from build123d import *

# Parameters (mm, degrees)
SKETCH_1_W                   = 15.864971157
SKETCH_1_H                   = 12.5
EXTRUDE_1_DEPTH              = 10
EXTRUDE_2_DEPTH              = 7.5
EXTRUDE_3_DEPTH              = 7.5
HOLE_WIZARD_M3_1_D           = 3.3
HOLE_WIZARD_M3_1_DEPTH       = 9.8
HOLE_WIZARD_M3_1_CBORE_D     = 6
HOLE_WIZARD_M3_1_CBORE_DEPTH = 0.8
HOLE_WIZARD_M3_1_TIP         = 0.991420021
HOLE_WIZARD_M3_2_D           = 3.4
HOLE_WIZARD_M3_2_CBORE_D     = 6.5
HOLE_WIZARD_M3_2_CBORE_DEPTH = 3.5
FILLET_1_R                   = 3
CHAMFER_1_SIZE               = 1.5
FILLET_2_R                   = 2


with BuildPart() as part:
    # 草图1 → 凸台-拉伸1 (new body)
    with BuildSketch(Plane(origin=(0, 5, 0), x_dir=(1, 0, 0), z_dir=(0, 1, 0))):
        with Locations((16.367514422, -6.25)):
            Rectangle(SKETCH_1_W, SKETCH_1_H)
    extrude(amount=-EXTRUDE_1_DEPTH)

    # 草图2 → 凸台-拉伸2 (add)
    with BuildSketch(Plane(origin=(0, 0, 0), x_dir=(-1, 0, 0), z_dir=(0, 0, -1))):
        with BuildLine():
            Line((-8.435028843, -5), (-18.435028843, -5))
            Line((-18.435028843, -5), (-18.435028843, -13.435028843))
            ThreePointArc((-18.435028843, -13.435028843), (-13.435028843, -18.435028843), (-8.435028843, -13.435028843))
            Line((-8.435028843, -13.435028843), (-8.435028843, -5))
        make_face()
    extrude(amount=-EXTRUDE_2_DEPTH)

    # 草图3 → 凸台-拉伸3 (add)
    with BuildSketch(Plane(origin=(0, 0, 0), x_dir=(-1, 0, 0), z_dir=(0, 0, -1))):
        with BuildLine():
            Line((-8.435028843, 5), (-8.435028843, 13.435028843))
            ThreePointArc((-8.435028843, 13.435028843), (-13.435028843, 18.435028843), (-18.435028843, 13.435028843))
            Line((-18.435028843, 13.435028843), (-18.435028843, 5))
            Line((-18.435028843, 5), (-8.435028843, 5))
        make_face()
    extrude(amount=-EXTRUDE_3_DEPTH)

    # M3 六角头机械螺钉的柱形沉头孔1
    with Locations(Plane(origin=(24.3, 0, 0), x_dir=(0, 0, -1), z_dir=(1, 0, 0))):
        with Locations((-7.5, 0)):
            CounterBoreHole(HOLE_WIZARD_M3_1_D / 2, HOLE_WIZARD_M3_1_CBORE_D / 2, HOLE_WIZARD_M3_1_CBORE_DEPTH, depth=HOLE_WIZARD_M3_1_DEPTH)
            with Locations((0, 0, -(HOLE_WIZARD_M3_1_DEPTH + HOLE_WIZARD_M3_1_TIP / 2))):  # 118° drill point
                Cone(0, HOLE_WIZARD_M3_1_D / 2, HOLE_WIZARD_M3_1_TIP, mode=Mode.SUBTRACT)

    # M3 六角头机械螺钉的柱形沉头孔2 (through all)
    with Locations(Plane.XY.offset(7.5)):
        with Locations((13.435028843, 13.435028843), (13.435028843, -13.435028843)):
            CounterBoreHole(HOLE_WIZARD_M3_2_D / 2, HOLE_WIZARD_M3_2_CBORE_D / 2, HOLE_WIZARD_M3_2_CBORE_DEPTH)

    # 圆角1
    fillet_1_edges = [part.edges().sort_by_distance(p)[0] for p in [
        (8.435028843, -5, 10),
        (8.435028843, 5, 10),
    ]]
    fillet(fillet_1_edges, radius=FILLET_1_R)

    # 倒角1
    chamfer_1_edges = [part.edges().sort_by_distance(p)[0] for p in [
        (8.435028843, 0, 12.5),
        (17.867514421, 5, 12.5),
        (17.867514421, -5, 12.5),
        (9.313708499, 4.121320344, 12.5),
        (9.313708499, -4.121320344, 12.5),
    ]]
    chamfer(chamfer_1_edges, length=CHAMFER_1_SIZE)

    # 圆角2
    fillet_2_edges = [part.edges().sort_by_distance(p)[0] for p in [
        (18.435028843, -5, 3.75),
        (18.435028843, 5, 3.75),
    ]]
    fillet(fillet_2_edges, radius=FILLET_2_R)


solid = part.part
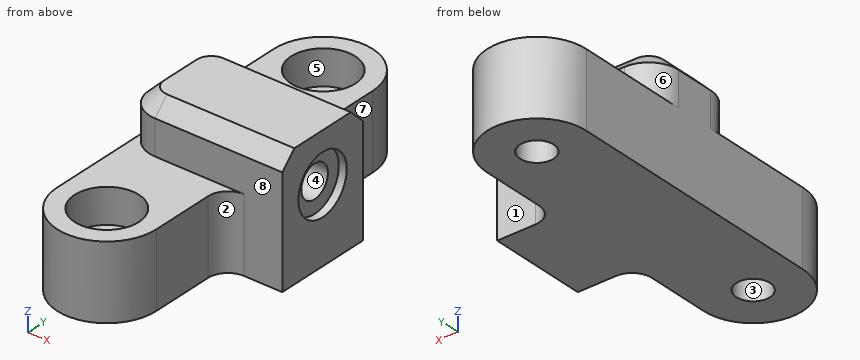
Here's how the part is built. I have some questions about the finished solid (model axes, mm). Face numbers are marked on the shaded views. A direction names the side the tool comes from. Give positions to 0.01 mm unless a question says otherwise; leave off trailing zeros. Order: outer loops, then holes, each group sorted by start corner. A loop starts at its lowest first (then second) coordinate and runs counter-clockwise, first axis right, second up. Notation, with made-up numbers: M -4,73.5 L 51,73.5 A23 ccw 51,100.5 Z; hole C -24.75,-37 d5. An arc over 180 degrees is marked long. Answer as a JSON object with one key per item and string values. Group by question number.
1) Please list where these lines run through material, in increasing order: L1, parallel to X at y = -13.5, z = 7.25; L2, parallel to Y at x = 16, z = 5.75; L3, parallel to Y at x = 23.8, z = 7.5. Write a range as [from, to].
2) Suppose I cut it at B-B, the plane z = 2.25. Write out the boundary of the cut face in (x, y), plus the area to 3 significant figures.
3) Suppose I cut it at A-A, the plane x = 21.75. Write out the boundary of the cut face in (y, z), plus the area to 3 significant figures.
4) Suppose I cut it at D-D, the plane x = 13. Write out the boundary of the cut face in (y, z), plus the area to 3 significant figures.
5) Suppose I cut it at C-C, the plane y = -14. Write out the boundary of the cut face in (x, z), plus the area to 3 significant figures.
6) We'd pull the mould along Y, two halves only. Please class the marked faces 1, 2 and 3: pulls with the +Y half, pulls with the -Y half, needs draft (parallel to the pull), parting line crosses it, or undercut.
7) On a 3-axis mill with a long thin cutter (end or side, diameter ignored), from which of +Z, -Z, +X, -X, +Y, -Y can I reach the whole of each face in a straight line? I mean the marked faces 4, 5, 6, 7 and 8. Say none if no direction works.
8) I'm going to push flat-ended pins straight in: pin 1 Ø5 at (y, z) = (8.5, 4) entering from +X; pin 2 Ø7 at (y, z) = (-11, 2.5) entering from +X (3 decimals); pin 3 Ø5 at (x, y) = (14.5, -13.5) entering from +Z. Where does each tip first touch, or does it pass through?
Results found:
{
 "1": {"L1": "[8.44, 10.19], [16.68, 18.43]", "L2": "[-17.73, -15.43], [-11.44, 11.44], [15.43, 17.73]", "L3": "[-5, -3], [3, 5]"},
 "2": {"outline": "M 8.44,-13.44 A5 ccw 18.44,-13.44 L 18.44,-7 A2 cw 20.44,-5 L 24.3,-5 L 24.3,5 L 20.44,5 A2 cw 18.44,7 L 18.44,13.44 A5 ccw 8.44,13.44 Z; hole C 13.44,-13.44 d3.4; hole C 13.44,13.44 d3.4", "area": "389 mm²"},
 "3": {"outline": "M -5,0 L 5,0 L 5,11 L 3.5,12.5 L -3.5,12.5 L -5,11 Z; hole C 0,7.5 d3.3", "area": "114 mm²"},
 "4": {"outline": "M -18.42,0 L -15.08,0 L -15.08,4 L -16.66,4 L -16.66,7.5 L -18.42,7.5 Z; M -11.79,0 L 11.79,0 L 11.79,4 L 10.21,4 L 10.21,7.5 L 5,7.5 L 5,11 L 3.5,12.5 L -3.5,12.5 L -5,11 L -5,7.5 L -10.21,7.5 L -10.21,4 L -11.79,4 Z; M 15.08,0 L 18.42,0 L 18.42,7.5 L 16.66,7.5 L 16.66,4 L 15.08,4 Z", "area": "253 mm²"},
 "5": {"outline": "M 8.47,0 L 11.83,0 L 11.83,4 L 10.23,4 L 10.23,7.5 L 8.47,7.5 Z; M 15.04,0 L 18.4,0 L 18.4,7.5 L 16.64,7.5 L 16.64,4 L 15.04,4 Z", "area": "39.3 mm²"},
 "6": {"face 1": "pulls with the +Y half", "face 2": "pulls with the -Y half", "face 3": "undercut"},
 "7": {"face 4": "+X", "face 5": "+Z", "face 6": "+Z, -X, +Y", "face 7": "+Z, -Z, +X, +Y", "face 8": "+Z, +X, -Y"},
 "8": {"pin 1": "x = 18.7", "pin 2": "x = 18.435", "pin 3": "z = 7.5"}
}
